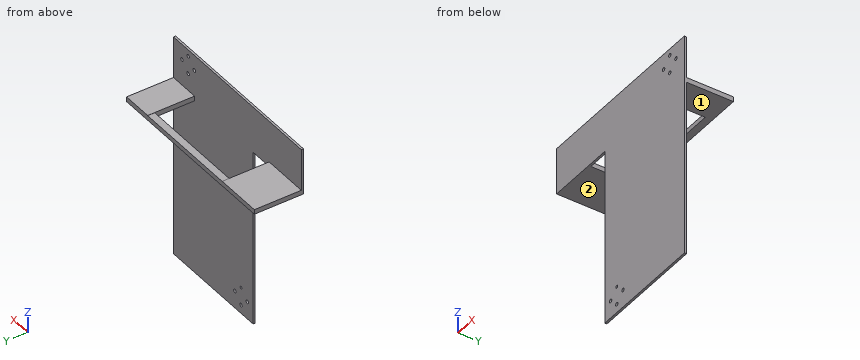
Autodesk Inventor part; units mm, degrees
ref_plane "YZ Plane" through (0, 0, 0) normal (1, 0, 0) x (0, 1, 0)
ref_plane "XZ Plane" through (0, 0, 0) normal (0, 1, 0) x (-1, 0, 0)
ref_plane "XY Plane" through (0, 0, 0) normal (0, 0, 1) x (1, 0, 0)
sketch "Sketch1" plane through (0, 0, 0) normal (0, 1, 0) x (-1, 0, 0)
  line L0 (0, 0) -> (177.8, 0)
  line L1 (177.8, 0) -> (177.8, -243.078)
  line L2 (177.8, -243.078) -> (0, -243.078)
  line L3 (0, -243.078) -> (0, 0)
  dimension "d0" = 243.078
  dimension "d1" = 177.8
extrude "Extrusion1" add sketch "Sketch1" along normal blind 2.286
sketch "Sketch2" plane through (0, 2.286, 0) normal (0, 1, 0) x (1, 0, 0)
  circle A0 centre (-75.024, 26.7891) radius 1.905
  circle A1 centre (-65.245, 17.0101) radius 1.905
  circle A2 centre (-75.024, 7.2311) radius 1.905
  circle A3 centre (-84.803, 17.0101) radius 1.905
  dimension "d7" = 3.81
  dimension "d8" = 3.81
  dimension "d9" = 3.81
  dimension "d10" = 3.81
extrude "Extrusion2" cut sketch "Sketch2" against normal blind 5.461
sketch "Sketch4" plane through (0, 2.286, 0) normal (0, 1, 0) x (1, 0, 0)
  line L0 (0, 0) -> (-177.8, 0)
  line L1 (-177.8, 0) -> (-177.8, 50.8)
  line L2 (-177.8, 50.8) -> (0, 50.8)
  line L3 (0, 50.8) -> (0, 45.5143)
  line L4 (0, 0) -> (0, 243.078)
  line L5 (0, 45.5143) -> (-177.8, 45.5143)
  line L6 (-85.237, 50.8) -> (-85.237, 45.5143)
  point P0 (0, 188.468)
  dimension "d16" = 50.8
extrude "Extrusion4" add sketch "Sketch4" along normal blind 50.8 contours L5 L6 L2 L3
sketch "Sketch6" plane through (-177.8, 0, -243.078) normal (-1, 0, 0) x (0, 0, 1)
  line L0 (243.078, 0) -> (0, 0)
  line L1 (0, 2.286) -> (243.078, 2.286)
  line L2 (243.078, 0) -> (192.4335, 0)
  line L3 (192.4335, 0) -> (192.4335, 2.286)
  line L4 (192.4335, 2.286) -> (243.078, 2.286)
  line L5 (243.078, 2.286) -> (243.078, 0)
  point P0 (3.81, 2.286)
  point P1 (243.078, 2.286)
  point P2 (192.4335, 0)
  dimension "d28" = 243.078
extrude "Extrusion6" add sketch "Sketch6" along normal blind 76.2
sketch "Sketch7" plane through (0, 2.286, 0) normal (0, 1, 0) x (1, 0, 0)
  line L0 (-177.8, 50.6445) -> (-254, 50.6445)
  line L1 (-254, 50.6445) -> (-203.1257, 50.6445)
  line L2 (-203.1257, 50.6445) -> (-203.1257, 45.5645)
  line L3 (-203.1257, 45.5645) -> (-254, 45.5645)
  line L4 (-254, 45.5645) -> (-254, 50.6445)
  point P0 (0, 0)
  dimension "d31" = 5.08
extrude "Extrusion7" add sketch "Sketch7" along normal blind 50.8
sketch "Sketch8" plane through (0, 2.286, -50.8) normal (0, 0, -1) x (-1, 0, 0)
  line L0 (0, 50.8) -> (85.237, 50.8)
  line L1 (203.1257, 0) -> (203.1257, 50.8)
  line L2 (85.237, 50.8) -> (203.1257, 50.8)
  line L3 (203.1257, 50.8) -> (203.1257, 43.18)
  line L4 (203.1257, 43.18) -> (85.237, 43.18)
  line L5 (85.237, 43.18) -> (85.237, 50.8)
  point P0 (0, -2.286)
  dimension "d34" = 50.8
  dimension "d35" = 7.62
extrude "Extrusion8" add sketch "Sketch8" against normal blind 5.08
sketch "Sketch10" plane through (0, 53.086, 0) normal (0, 1, 0) x (1, 0, 0)
  line L0 (0, 0) -> (-254, 0)
  line L1 (0, 188.468) -> (-177.8, 188.468)
  line L2 (-51.904, 0) -> (0, 0)
  line L3 (0, 0) -> (0, 188.468)
  line L4 (0, 188.468) -> (-51.904, 188.468)
  line L5 (-51.904, 188.468) -> (-51.904, 0)
  line L6 (0, 243.078) -> (-177.8, 243.078)
  line L7 (-51.904, 188.468) -> (0, 188.468)
  line L8 (0, 188.468) -> (0, 243.078)
  line L9 (0, 243.078) -> (-51.904, 243.078)
  line L10 (-51.904, 243.078) -> (-51.904, 188.468)
extrude "Extrusion9" cut sketch "Sketch10" against normal blind 87.3125
sketch "Sketch11" plane through (0, 2.286, 0) normal (0, 1, 0) x (1, 0, 0)
  line L0 (-177.8, 243.078) -> (-177.8, 50.6445)
  line L1 (-177.8, 243.078) -> (-139.7, 243.078)
  line L2 (-139.7, 243.078) -> (-139.7, 204.978)
  line L3 (-139.7, 204.978) -> (-177.8, 204.978)
  line L4 (-177.8, 204.978) -> (-177.8, 243.078)
  circle A0 centre (-158.75, 224.028) radius 9.779
  circle A1 centre (-168.529, 224.028) radius 1.905
  circle A2 centre (-158.75, 233.807) radius 1.905
  circle A3 centre (-158.75, 214.249) radius 1.4605
  circle A4 centre (-148.971, 224.028) radius 1.905
  point P0 (0, 0)
  dimension "d40" = 38.1
  dimension "d41" = 38.1
  dimension "d42" = 19.558
  dimension "d43" = 3.81
  dimension "d44" = 3.81
  dimension "d45" = 2.921
  dimension "d46" = 3.81
extrude "Extrusion10" cut sketch "Sketch11" against normal blind 25.4 contours A0 A4 | A0 A4 | A2 A0 | A0 A2 | A3 A0 | A0 A3 | A1 A0 | A0 A1
properties part number "Plate"
Build history of the part. All positions in model axes, mm. Face numbers are marked on the shaded views. A direction names the side the tool comes from. Give positions to 0.01 mm unless a question says otherwise; leave off trailing zeros. Order: outer loops, then holes, each group sorted by start corner. A loop starts at its lowest first (then second) coordinate and runs counter-clockwise, first axis right, second up. Notation, with made-up numbers: M 32.25,30.5 L 77.25,30.5 A18 cw 77.25,60.5 Z; hole C -35.5,32.5 d7. An arc over 180 degrees is marked long. Put each result on its own line as item: value.
Item 1: Wall check: probe 1 along Z at (x, y) = (-158.75, 1.55); probe 2 along Z at (x, y) = (-223, 44); probe 3 along Y at (x, z) = (-157, -93). Give the ranges that are in metal, low to high.
Results are:
probe 1: -243.08 to -235.71, -231.9 to -215.71, -212.79 to 0
probe 2: -50.64 to -45.56
probe 3: 0 to 2.29
Item 2: Cut at B-B on y = 31.5. Write the cut outline in (x, z), then the cut area to 3 significant figures.
Results are:
outline: M -254,-50.64 L -203.13,-50.64 L -203.13,-45.56 L -254,-45.56 Z; M -85.24,-50.8 L -51.9,-50.8 L -51.9,-45.51 L -85.24,-45.51 Z
area: 435 mm2
Item 3: Cut at C-C on x = -227.5. Write the cut outline in (y, z).
Results are:
outline: M 0,-50.64 L 53.09,-50.64 L 53.09,-45.56 L 2.29,-45.56 L 2.29,0 L 0,0 Z
Item 4: Which spindle directions (+Z, -Z, +X, -X, +Y, -Y) get a long thin tool onto all of the face, cutting with end or side? Do the marked faces 1 and 2. Say none if no direction does.
Results are:
face 1: -Z, +X, -X, +Y
face 2: -Z, -X, +Y, -Y
Item 5: Cut at A-A on x = -90. Write the cut outline in (y, z), then the cut area to 3 significant figures.
Results are:
outline: M 0,-243.08 L 2.29,-243.08 L 2.29,0 L 0,0 Z; M 45.47,-50.8 L 53.09,-50.8 L 53.09,-45.72 L 45.47,-45.72 Z
area: 594 mm2
Item 6: Drop flat-ended pins along their axis: pin 1 Ø12 at (x, z) = (-100.5, -91.5) entering from +Y; pin 2 Ø3.5 at (x, z) = (-148.971, -224.028) entering from +Y; pin 3 Ø1.8 at (y, z) = (1, -104.5) entering from -X; pin 4 Ø10 at (x, y) = (-73.5, 18.5) entering from +Z. Give the stop position or say it passes through.
Results are:
pin 1: y = 2.29
pin 2: through
pin 3: x = -177.8
pin 4: z = -45.51
Item 7: Cut at D-D on z = -173. Write the cut outline in (x, y), then the cut area to 3 significant figures.
Results are:
outline: M -177.8,0 L -51.9,0 L -51.9,2.29 L -177.8,2.29 Z
area: 288 mm2
